Build history of the part. All positions in model axes, mm. Give positions to 0.01 mm unless a question says otherwise; leave off trailing zeros. Loops run counter-clockwise (first coordinate to the right, second up) from the corner with the lowest first, then second, coordinate; pieces in that order, holes last. Notation, with made-up numbers: (48, -11.75) -> (80, -11.75) arc R19 ccw to (80, 23.25) -> close; hole circle Ø2 at (12, -24). An arc over 180 degrees is marked (long way). Answer as a JSON object with one key per item and string values. Group by question number.
Autodesk Fusion 360 part; units mm, degrees
sketch "Cuadrado 100x100" plane through (0, 0, 0) normal (0, 0, 1) x (1, 0, 0)
  line L0 (50, -50) -> (-50, -50)
  line L1 (-50, -50) -> (-50, 50)
  line L2 (-50, 50) -> (50, 50)
  line L3 (50, 50) -> (50, -50)
  line L4 (50, -50) -> (-50, 50) construction
  line L5 (-50, -50) -> (50, 50) construction
  dimension "d1" = 100
sketch "Sketch1" plane through (0, 0, 0) normal (0, 0, 1) x (1, 0, 0) in component "plate"
  line L0 (22.5, 22.5) -> (-22.5, 22.5)
  line L1 (-22.5, 22.5) -> (-22.5, -22.5)
  line L2 (-22.5, -22.5) -> (22.5, -22.5)
  line L3 (22.5, -22.5) -> (22.5, 22.5)
  line L4 (22.5, 22.5) -> (-22.5, -22.5) construction
  line L5 (-22.5, 22.5) -> (22.5, -22.5) construction
  line L6 (15.5, 15.5) -> (-15.5, 15.5)
  line L7 (-15.5, 15.5) -> (-15.5, -15.5)
  line L8 (-15.5, -15.5) -> (15.5, -15.5)
  line L9 (15.5, -15.5) -> (15.5, 15.5)
  line L10 (122.5, -50) -> (22.5, -50)
  line L11 (22.5, -50) -> (22.5, 50)
  line L12 (22.5, 50) -> (122.5, 50)
  line L13 (122.5, 50) -> (122.5, -50)
  line L14 (122.5, -50) -> (22.5, 50) construction
  line L15 (22.5, -50) -> (122.5, 50) construction
  line L16 (110.7039, 38.2039) -> (34.2961, 38.2039)
  line L17 (34.2961, 38.2039) -> (34.2961, -38.2039)
  line L18 (34.2961, -38.2039) -> (110.7039, -38.2039)
  line L19 (110.7039, -38.2039) -> (110.7039, 38.2039)
  line L20 (72.5, 0) -> (22.5, 0) construction
  point P0 (72.5, 0)
  point P1 (72.5, 0)
  dimension "d59" = 45
  dimension "d60" = 31
  dimension "d62" = 100
extrude "Extrude1" add sketch "Sketch1" against normal blind 6 contours L0 L1 L2 L3 L11 | L3 L10 L11 L12 L13 | L6 L7 L8 L9 in component "plate"
fillet "Fillet1" radius 2 14 edges at (-22.5, 22.5, -3) (-22.5, -22.5, -3) (22.5, 22.5, -3) (22.5, 50, -3) (122.5, 50, -3) (122.5, -50, -3) (22.5, -22.5, -3) (22.5, -50, -3) (22.5, -22.5, -3) (22.5, -50, -3) (34.2961, 38.2039, -3) (110.7039, 38.2039, -3) (110.7039, -38.2039, -3) (34.2961, -38.2039, -3) in component "plate"
chamfer "Chamfer1" distance 0.5 angle 45 48 edges at (122.5, 0, 0) (121.9142, -49.4142, 0) (72.5, -50, 0) (23.0858, -49.4142, 0) (22.5, -36.25, 0) (21.9142, -23.0858, 0) (0, -22.5, 0) (-21.9142, -21.9142, 0) (-22.5, 0, 0) (-21.9142, 21.9142, 0) (0, 22.5, 0) (21.9142, 23.0858, 0) (22.5, 36.25, 0) (23.0858, 49.4142, 0) (72.5, 50, 0) (121.9142, 49.4142, 0) (122.5, 0, -6) (121.9142, 49.4142, -6) (72.5, 50, -6) (23.0858, 49.4142, -6) (22.5, 36.25, -6) (21.9142, 23.0858, -6) (0, 22.5, -6) (-21.9142, 21.9142, -6) (-22.5, 0, -6) (-21.9142, -21.9142, -6) (0, -22.5, -6) (21.9142, -23.0858, -6) (22.5, -36.25, -6) (23.0858, -49.4142, -6) (72.5, -50, -6) (121.9142, -49.4142, -6) (34.8819, 37.6181, -6) (34.2961, 0, -6) (34.8819, -37.6181, -6) (72.5, -38.2039, -6) (110.1181, -37.6181, -6) (110.7039, 0, -6) (110.1181, 37.6181, -6) (72.5, 38.2039, -6) (110.1181, 37.6181, 0) (110.7039, 0, 0) (110.1181, -37.6181, 0) (72.5, -38.2039, 0) (34.8819, -37.6181, 0) (34.2961, 0, 0) (34.8819, 37.6181, 0) (72.5, 38.2039, 0) in component "plate"
hole "Hole1" at (15.5, 15.5, 0) at (-15.5, 15.5, 0) at (-15.5, -15.5, 0) at (15.5, -15.5, 0) direction (0, 0, -1) diameter 3 end through all countersink diameter 6 countersink angle 90 in component "plate"
component "plate" placed x (1, 0, 0) y (0, 1, 0) z (0, 0, 1) at (0, 0, 0)
equation "offsetI3dDiam = 0.2 mm"
equation "offsetI3dRad = offsetI3dDiam / 2"
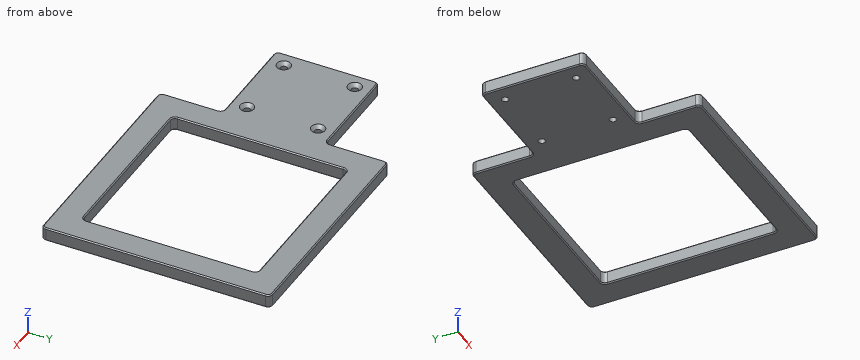
(1) Saw through at D-D on x = 15.5. List the corners of the cut face in (y, z), plus the area to 3 significant figures.
(2) Saw through at B-B on z = -3.55. List the corners of the cut face in (x, y).
(3) Saw through at C-C on y = -15.5. List the corners of the cut face in (x, z), plus the area to 3 significant figures.
(4) Saw through at A-A on y = 27.5. List the corners of the cut face in (x, z).
(5) Pin check, flat tips, straight feed: pin 1 (2.5 mm diameter, centred on y = -35, z = -2, fed in from -X); pin 2 (3.5 mm diameter, centred on x = 15.5, y = 15.5, fed in from +Z). Stop position of each tip, or through.
(6) Probe line 1 along Y through (x, z) = (-15.5, -3); line 2 along X through (y, z) = (15.5, -5); line 3 along Y through (x, z) = (55, -3.5). List the from-to ranges inside material, lowest first. Write a range as [from, to].
Calculated:
{
 "1": {"outline": "(-22.5, -5.5) -> (-22, -6) -> (-17, -6) -> (-17, -1.5) -> (-18.5, 0) -> (-22, 0) -> (-22.5, -0.5) -> close; (-14, -6) -> (14, -6) -> (14, -1.5) -> (12.5, 0) -> (-12.5, 0) -> (-14, -1.5) -> close; (17, -6) -> (22, -6) -> (22.5, -5.5) -> (22.5, -0.5) -> (22, 0) -> (18.5, 0) -> (17, -1.5) -> close", "area": "229 mm^2"},
 "2": {"outline": "(-22.5, -20.5) arc R2 ccw to (-20.5, -22.5) -> (20.5, -22.5) arc R2 cw to (22.5, -24.5) -> (22.5, -48) arc R2 ccw to (24.5, -50) -> (120.5, -50) arc R2 ccw to (122.5, -48) -> (122.5, 48) arc R2 ccw to (120.5, 50) -> (24.5, 50) arc R2 ccw to (22.5, 48) -> (22.5, 24.5) arc R2 cw to (20.5, 22.5) -> (-20.5, 22.5) arc R2 ccw to (-22.5, 20.5) -> close; hole circle Ø3 at (-15.5, -15.5); hole circle Ø3 at (-15.5, 15.5); hole circle Ø3 at (15.5, -15.5); hole circle Ø3 at (15.5, 15.5); hole (34.3, -36.2) arc R2 ccw to (36.3, -38.2) -> (108.7, -38.2) arc R2 ccw to (110.7, -36.2) -> (110.7, 36.2) arc R2 ccw to (108.7, 38.2) -> (36.3, 38.2) arc R2 ccw to (34.3, 36.2) -> close"},
 "3": {"outline": "(-22.5, -5.5) -> (-22, -6) -> (-17, -6) -> (-17, -1.5) -> (-18.5, 0) -> (-22, 0) -> (-22.5, -0.5) -> close; (-14, -6) -> (14, -6) -> (14, -1.5) -> (12.5, 0) -> (-12.5, 0) -> (-14, -1.5) -> close; (17, -6) -> (33.8, -6) -> (34.3, -5.5) -> (34.3, -0.5) -> (33.8, 0) -> (18.5, 0) -> (17, -1.5) -> close; (110.7, -5.5) -> (111.2, -6) -> (122, -6) -> (122.5, -5.5) -> (122.5, -0.5) -> (122, 0) -> (111.2, 0) -> (110.7, -0.5) -> close", "area": "370 mm^2"},
 "4": {"outline": "(22.5, -5.5) -> (23, -6) -> (33.8, -6) -> (34.3, -5.5) -> (34.3, -0.5) -> (33.8, 0) -> (23, 0) -> (22.5, -0.5) -> close; (110.7, -5.5) -> (111.2, -6) -> (122, -6) -> (122.5, -5.5) -> (122.5, -0.5) -> (122, 0) -> (111.2, 0) -> (110.7, -0.5) -> close"},
 "5": {"pin 1": "stops at x = 22.5", "pin 2": "stops at z = -1.25"},
 "6": {"line 1": "y = [-22.5, -17], [-14, 14], [17, 22.5]", "line 2": "x = [-22.5, -17], [-14, 14], [17, 34.3], [110.7, 122.5]", "line 3": "y = [-50, -38.2], [38.2, 50]"}
}
